Work out the finished part from the listing and answer in its coordinate system (mm). Give positions to 0.01 mm unless a question says otherwise; leave off trailing zeros. Loops run counter-clockwise (first coordinate to the right, second up) from the corner with the lowest first, then second, coordinate; pieces in that order, holes last.
from build123d import *

# Parameters (mm, degrees)
CROQUIS1_W              = 88
CROQUIS1_H              = 88
CROQUIS1_R              = 1.5
SALIENTE_EXTRUIR1_DEPTH = 15


with BuildPart() as part:
    # Croquis1 → Saliente-Extruir1 (new body)
    with BuildSketch(Plane(origin=(0, 0, 0), x_dir=(0, 0, -1), z_dir=(1, 0, 0))):
        with Locations((44, 44)):
            Rectangle(CROQUIS1_W, CROQUIS1_H)
        with Locations((5, 82)):
            Circle(CROQUIS1_R, mode=Mode.SUBTRACT)
        with Locations((29, 82)):
            Circle(CROQUIS1_R, mode=Mode.SUBTRACT)
        with Locations((29, 64)):
            Circle(CROQUIS1_R, mode=Mode.SUBTRACT)
        with Locations((5, 64)):
            Circle(CROQUIS1_R, mode=Mode.SUBTRACT)
        with Locations(Location((59, 64, 0), (0, 0, 180))):
            Circle(CROQUIS1_R, mode=Mode.SUBTRACT)
        with Locations(Location((59, 82, 0), (0, 0, 180))):
            Circle(CROQUIS1_R, mode=Mode.SUBTRACT)
        with Locations(Location((83, 64, 0), (0, 0, 180))):
            Circle(CROQUIS1_R, mode=Mode.SUBTRACT)
        with Locations(Location((83, 82, 0), (0, 0, 180))):
            Circle(CROQUIS1_R, mode=Mode.SUBTRACT)
        with Locations((83, 24)):
            Circle(CROQUIS1_R, mode=Mode.SUBTRACT)
        with Locations((59, 24)):
            Circle(CROQUIS1_R, mode=Mode.SUBTRACT)
        with Locations((83, 6)):
            Circle(CROQUIS1_R, mode=Mode.SUBTRACT)
        with Locations((59, 6)):
            Circle(CROQUIS1_R, mode=Mode.SUBTRACT)
        with Locations(Location((29, 24, 0), (0, 0, 180))):
            Circle(CROQUIS1_R, mode=Mode.SUBTRACT)
        with Locations(Location((5, 24, 0), (0, 0, 180))):
            Circle(CROQUIS1_R, mode=Mode.SUBTRACT)
        with Locations(Location((29, 6, 0), (0, 0, 180))):
            Circle(CROQUIS1_R, mode=Mode.SUBTRACT)
        with Locations(Location((5, 6, 0), (0, 0, 180))):
            Circle(CROQUIS1_R, mode=Mode.SUBTRACT)
        with Locations((25.2, 44)):
            Circle(CROQUIS1_R, mode=Mode.SUBTRACT)
        with Locations((62.8, 44)):
            Circle(CROQUIS1_R, mode=Mode.SUBTRACT)
    extrude(amount=SALIENTE_EXTRUIR1_DEPTH)


solid = part.part
Item 1: Find section D-D, the plane z = -59. Write down the section's boundary in (x, y), plus the area to 3 significant figures.
Item 2: Determine the mould class of faces 1 (the face through (7, 88, -43)), 2 (the face through (7.395, 83.487, -28.805)), 3 (the face through (15, 45, -43)) for opening direction Y: released by +Y, released by -Y, zero draft, split by the parting line, or undercut.
Item 3: Find section A-A, the plane y = 44. Write down the section's boundary in (x, z).
Item 4: Consider line 1 (Z direction, x = 3.25, y = 64); line 2 (Y direction, x = 11, z = -59); line 3 (Y direction, x = 11, z = -25.2). Determine where each line is inside the solid, lowest interval first.
Item 5: Find section B-B, the plane x = 11.75. Give the number of separate pieces and of enclosed holes in the cut face, plus the area to 3 significant figures.
Item 6: Find section C-C, the plane y = 82. Write down the section's boundary in (x, z), plus the area to 3 significant figures.
Ans:
1. outline: (0, 0) - (15, 0) - (15, 4.5) - (0, 4.5) - close; (0, 7.5) - (15, 7.5) - (15, 22.5) - (0, 22.5) - close; (0, 25.5) - (15, 25.5) - (15, 62.5) - (0, 62.5) - close; (0, 65.5) - (15, 65.5) - (15, 80.5) - (0, 80.5) - close; (0, 83.5) - (15, 83.5) - (15, 88) - (0, 88) - close
1. area: 1,140 mm2
2. face 1: released by +Y
2. face 2: undercut
2. face 3: zero draft
3. outline: (0, -88) - (15, -88) - (15, -64.3) - (0, -64.3) - close; (0, -61.3) - (15, -61.3) - (15, -26.7) - (0, -26.7) - close; (0, -23.7) - (15, -23.7) - (15, 0) - (0, 0) - close
4. line 1: z = -88 to -84.5, -81.5 to -60.5, -57.5 to -30.5, -27.5 to -6.5, -3.5 to 0
4. line 2: y = 0 to 4.5, 7.5 to 22.5, 25.5 to 62.5, 65.5 to 80.5, 83.5 to 88
4. line 3: y = 0 to 42.5, 45.5 to 88
5. separate pieces: 1
5. enclosed holes: 18
5. area: 7,620 mm2
6. outline: (0, -88) - (15, -88) - (15, -84.5) - (0, -84.5) - close; (0, -81.5) - (15, -81.5) - (15, -60.5) - (0, -60.5) - close; (0, -57.5) - (15, -57.5) - (15, -30.5) - (0, -30.5) - close; (0, -27.5) - (15, -27.5) - (15, -6.5) - (0, -6.5) - close; (0, -3.5) - (15, -3.5) - (15, 0) - (0, 0) - close
6. area: 1,140 mm2
